```python
from build123d import *

# Parameters (mm, degrees)
CROQUIS1_W              = 42.3
CROQUIS1_H              = 42.3
SALIENTE_EXTRUIR1_DEPTH = 12
CORTAR_EXTRUIR1_DEPTH   = 2
CHAFL_N1_SIZE           = 2
CROQUIS3_R              = 1.5
CORTAR_EXTRUIR2_DEPTH   = 10
CROQUIS4_R              = 12
CORTAR_EXTRUIR3_DEPTH   = 2
CROQUIS5_R              = 11
SALIENTE_EXTRUIR2_DEPTH = 4
CROQUIS6_R              = 3.5
CORTAR_EXTRUIR5_DEPTH   = 2
CROQUIS7_R              = 2.5
CORTAR_EXTRUIR6_DEPTH   = 13


with BuildPart() as part:
    # Croquis1 → Saliente-Extruir1 (new body)
    with BuildSketch(Plane(origin=(0, 0, 0), x_dir=(1, 0, 0), z_dir=(0, 1, 0))):
        Rectangle(CROQUIS1_W, CROQUIS1_H)
    extrude(amount=SALIENTE_EXTRUIR1_DEPTH)

    # Croquis2 → Cortar-Extruir1 (cut)
    with BuildSketch(Plane(origin=(0, 12, 0), x_dir=(1, 0, 0), z_dir=(0, 1, 0))):
        with BuildLine():
            Line((-21.15, 13.329572386), (-21.15, -13.329572386))
            ThreePointArc((-21.15, -13.329572386), (-17.67766953, -17.67766953), (-13.329572386, -21.15))
            Line((-13.329572386, -21.15), (13.329572386, -21.15))
            ThreePointArc((13.329572386, -21.15), (17.67766953, -17.67766953), (21.15, -13.329572386))
            Line((21.15, -13.329572386), (21.15, 13.329572386))
            ThreePointArc((21.15, 13.329572386), (17.67766953, 17.67766953), (13.329572386, 21.15))
            Line((13.329572386, 21.15), (-13.329572386, 21.15))
            ThreePointArc((-13.329572386, 21.15), (-17.67766953, 17.67766953), (-21.15, 13.329572386))
        make_face()
    extrude(amount=-CORTAR_EXTRUIR1_DEPTH, mode=Mode.SUBTRACT)

    # Chaflán1
    chafl_n1_edges = [part.edges().sort_by_distance(p)[0] for p in [
        (21.15, 6, 21.15),
        (-21.15, 6, 21.15),
        (-21.15, 6, -21.15),
        (21.15, 6, -21.15),
    ]]
    chamfer(chafl_n1_edges, length=CHAFL_N1_SIZE)

    # Croquis3 → Cortar-Extruir2 (cut)
    with BuildSketch(Plane.XZ):
        with Locations((-15.5, 15.5)):
            Circle(CROQUIS3_R)
        with Locations((-15.5, -15.5)):
            Circle(CROQUIS3_R)
        with Locations((15.5, -15.5)):
            Circle(CROQUIS3_R)
        with Locations((15.5, 15.5)):
            Circle(CROQUIS3_R)
    extrude(amount=-CORTAR_EXTRUIR2_DEPTH, mode=Mode.SUBTRACT)

    # Croquis4 → Cortar-Extruir3 (cut)
    with BuildSketch(Plane.XZ):
        Circle(CROQUIS4_R)
    extrude(amount=-CORTAR_EXTRUIR3_DEPTH, mode=Mode.SUBTRACT)

    # Croquis5 → Saliente-Extruir2 (add)
    with BuildSketch(Plane.XZ.offset(-2)):
        Circle(CROQUIS5_R)
    extrude(amount=SALIENTE_EXTRUIR2_DEPTH)

    # Croquis6 → Cortar-Extruir5 (cut)
    with BuildSketch(Plane.XZ.offset(2)):
        Circle(CROQUIS6_R)
    extrude(amount=-CORTAR_EXTRUIR5_DEPTH, mode=Mode.SUBTRACT)

    # Croquis7 → Cortar-Extruir6 (cut, through all)
    with BuildSketch(Plane.XZ):
        Circle(CROQUIS7_R)
    extrude(amount=-CORTAR_EXTRUIR6_DEPTH, mode=Mode.SUBTRACT)


solid = part.part
```
Verification items for the finished model (mm, model axes). A direction names the side the tool comes from. Coordinates: 2 decimals unless noted, no trailing zeros. Write each loop counter-clockwise with the first axis right and the second up, starting at its lowest first coordinate (ties: lowest second). Pieces come first, ordered by that corner, then holes. Notation, with made-up numbers: M 27.5,16 L 85.5,16 A26 ccw 85.5,47 Z; hole C 13.5,-12.5 d4. An arc over 180 degrees is marked long. One line per item, written item: value.
Item 1: Access from +Z, -Z, +X, -X, +Y, -Y to the whole of each face (thin tool, end or side, straight path). Record for faces 4 (the cylindrical face through (-11.99, 0.99, 0.53)), 5 (the flat face through (0, 10, -5)), 6 (the flat face through (-18, 12, 18)).
Check sheet entries:
face 4: -Y
face 5: +Y
face 6: +Z, -Z, +X, -X, +Y
Item 2: Mould release check, pull along Z, two halves, no side actions. Record for faces 1 (the cylindrical face through (-17, 4.93, -15.43)), 2 (the flat face through (20.2, 5.9, -20.1)), 3 (the flat face through (-3, -2, 3)): pulls with the +Z half, pulls with the -Z half, needs draft (parallel to the pull), parting line crosses it, or undercut.
Check sheet entries:
face 1: undercut
face 2: pulls with the -Z half
face 3: needs draft
Item 3: Section check D-D, the plane z = 15.5. Record the boundary of the cut face in (x, y).
Check sheet entries:
outline: M -21.15,0 L -17,0 L -17,10 L -19.62,10 L -19.62,12 L -21.15,12 Z; M -14,0 L 14,0 L 14,10 L -14,10 Z; M 17,0 L 21.15,0 L 21.15,12 L 19.62,12 L 19.62,10 L 17,10 Z
Item 4: Scan lines: line 1 along Z through (x, y) = (15.5, 4); line 2 along Z through (x, y) = (0, 1.45); line 3 along Z through (x, y) = (0, -1.35). Record each from-to range of solid material in increasing order.
Check sheet entries:
line 1: z = -21.15 to -17, -14 to 14, 17 to 21.15
line 2: z = -21.15 to -12, -11 to -2.5, 2.5 to 11, 12 to 21.15
line 3: z = -11 to -3.5, 3.5 to 11
Item 5: Gauge pin test, flat ends, axial feed: pin 1 Ø1 at (x, z) = (-11, 12) entering from -Y; pin 2 Ø12 at (x, z) = (-5, -14.5) entering from +Y. Record the tip position at first contact, or that the pin passes through.
Check sheet entries:
pin 1: stops at y = 0
pin 2: stops at y = 10
Item 6: Section check C-C, the plane y = 11.25. Record the boundary of the cut face in (x, z).
Check sheet entries:
outline: M -21.15,-19.15 L -19.15,-21.15 L -13.33,-21.15 A25 cw -21.15,-13.33 Z; M -21.15,13.33 A25 cw -13.33,21.15 L -19.15,21.15 L -21.15,19.15 Z; M 13.33,-21.15 L 19.15,-21.15 L 21.15,-19.15 L 21.15,-13.33 A25 cw Z; M 13.33,21.15 A25 cw 21.15,13.33 L 21.15,19.15 L 19.15,21.15 Z
Item 7: Section check A-A, the plane y = 7. Record the boundary of the cut face in (x, z), plus the area to 3 significant figures.
Check sheet entries:
outline: M -21.15,-19.15 L -19.15,-21.15 L 19.15,-21.15 L 21.15,-19.15 L 21.15,19.15 L 19.15,21.15 L -19.15,21.15 L -21.15,19.15 Z; hole C -15.5,-15.5 d3; hole C -15.5,15.5 d3; hole C 0,0 d5; hole C 15.5,-15.5 d3; hole C 15.5,15.5 d3
area: 1,730 mm^2
Item 8: Section check B-B, the plane x = 0. Record the boundary of the cut face in (y, z).
Check sheet entries:
outline: M -2,-11 L 2,-11 L 2,-12 L 0,-12 L 0,-21.15 L 10,-21.15 L 10,-2.5 L 0,-2.5 L 0,-3.5 L -2,-3.5 Z; M -2,3.5 L 0,3.5 L 0,2.5 L 10,2.5 L 10,21.15 L 0,21.15 L 0,12 L 2,12 L 2,11 L -2,11 Z
